Geometry: final body of the model. Coordinates: model frame, mm. A direction names the side the tool comes from. Coordinates: 2 decimals unless noted, no trailing zeros. Order: outer loops, then holes, each group sorted by start corner. A loop starts at its lowest first (then second) coordinate and runs counter-clockwise, first axis right, second up. Notation, with made-up numbers: (5, 37.5) -> (59, 37.5) arc R22 ccw to (59, 70.5) -> close; hole circle Ø10 at (73.5, 81). An arc over 180 degrees is marked (long way). Answer in a Markdown table with one row per item. Add a question column.
1) Set-up query: faces 5 (the face through (9, 1.4, -10)), 6 (the face through (-9.22, 0.71, -10.03)). Return all of +Z, -Z, +X, -X, +Y, -Y with unobstructed straight access to the full face (end or side cutting, diameter ignored); none if empty.
2) Ray query, line 1 (X direction, y = 3.25, z = -9); line 2 (Z direction, x = 12, y = 2.9); line 3 (Z direction, x = 11.5, y = 4.45). Return the intervals inside material, ascending. Write a range as from..to.
3) Section query A-A on x = 0. Return the cut outline in (y, z), then the cut area to 3 significant figures.
4) Pull-direction query (Y, two-part tool) for faces 1 (the face through (0, 0, 0)), 2 (the face through (-9.167, 2.485, 13.124)), 3 (the face through (-9.15, 2.48, 8.1)), 4 (the face through (11.99, 0.71, -10.03)); classes: +Y half, -Y half, draft (parallel to the pull), parting line (faces both ways), or undercut.
5) Section query B-B on y = 4.45. Count the separate pieces of the cut face and the enclosed holes in it, then the cut area to 3 significant figures.
6) Section query C-C on z = 5.5. Return the cut outline in (x, y), then the cut area to 3 significant figures.
7) Contact query for flat-ended pins moving along their axis: P1, Ø3, axis at x = -18, y = 1.5, coming from the +Z side; P2, Ø3, axis at x = -4.5, y = 3.5, coming from the +Z side; P3, Ø2.5, axis at x = 10.61, z = 10.61, coming from the -Y side; P4, Ø6.5, axis at x = -10.5, z = -9.5, coming from the -Y side. Output: stop coordinate, or through.
Autodesk Inventor part; units mm, degrees
ref_plane "Work Plane1" through (0, 2.5, 0) normal (0, 1, 0) x (1, 0, 0)
ref_plane "YZ Plane" through (0, 0, 0) normal (1, 0, 0) x (0, 1, 0)
ref_plane "XZ Plane" through (0, 0, 0) normal (0, 1, 0) x (-1, 0, 0)
sketch "Sketch1" plane through (0, 0, 0) normal (0, 1, 0) x (-1, 0, 0)
  circle A0 centre (0, 0) radius 12.5
  circle A1 centre (12.5, 0) radius 2
  circle A2 centre (0, 12.5) radius 2
  circle A3 centre (-12.5, 0) radius 2
  circle A4 centre (0, -12.5) radius 2
  circle A5 centre (0, 0) radius 22.5
  dimension "d0" = 25
  dimension "d1" = 4
  dimension "d4" = 360
  dimension "d6" = 45
extrude "Extrusion1" add sketch "Sketch1" along normal blind 5 contours A1 A0 A4 A3 A2 | A5
chamfer "Chamfer1" distance 2 angle 45 4 edges at (-10.5, 5, 0) (2, 5, 12.5) (14.5, 5, 0) (2, 5, -12.5)
sketch "Sketch2" plane through (0, 5, 0) normal (0, 1, 0) x (1, 0, 0)
  circle A0 centre (0, 0) radius 15
  line L0 (0, 0) -> (-15, 0)
  line L1 (0, 0) -> (-10.6066, -10.6066)
  circle A1 centre (-10.6066, -10.6066) radius 1.5
  circle A2 centre (10.6066, -10.6066) radius 1.5
  circle A3 centre (10.6066, 10.6066) radius 1.5
  circle A4 centre (-10.6066, 10.6066) radius 1.5
  dimension "d12" = 30
  dimension "d13" = 45
  dimension "d14" = 3
  dimension "d17" = 360
extrude "Extrusion2" cut sketch "Sketch2" against normal blind 5 contours A3 A0 | A0 A3 | A2 A0 | A0 A2 | A4 A0 | A0 A4 | A1 A0 | A0 L1 A1 | A0 A1 L1
ref_plane "Work Plane1" through (0, 2.5, 0) normal (0, 1, 0) x (1, 0, 0)
sketch "Sketch4" plane through (0, 2.5, 0) normal (0, 1, 0) x (1, 0, 0)
  circle A0 centre (10.6066, 10.6066) radius 1.5
  circle A1 centre (10.6066, -10.6066) radius 1.5
  circle A2 centre (-10.6066, -10.6066) radius 1.5
  circle A3 centre (-10.6066, 10.6066) radius 1.5
  line L0 (13.4857, 8.8966) -> (10.5653, 7.2582)
  line L1 (10.5653, 7.2582) -> (7.6862, 8.9682)
  line L2 (7.6862, 8.9682) -> (7.7275, 12.3166)
  line L3 (7.7275, 12.3166) -> (10.6479, 13.955)
  line L4 (10.6479, 13.955) -> (13.527, 12.245)
  line L5 (13.527, 12.245) -> (13.4857, 8.8966)
  point P0 (0, 0)
  dimension "d28" = 5.8
extrude "Extrusion3" cut sketch "Sketch4" along normal mid plane 2.2 contours L0 L1 L2 L3 L4 L5
pattern_circular "Circular Pattern1" count 4 over 360 about axis through (0, 0, 0) along (0, 1, 0) of "Extrusion3"
properties part number "adaptador"
Result:
| question | item | result |
|---|---|---|
| 1 | face 5 | none |
| 1 | face 6 | +Y, -Y |
| 2 | line 1 | -20.62..-13.03, -8.19..7.69, 13.49..20.62 |
| 2 | line 2 | -19.03..-13.15, -8.06..-1.94, 1.94..7.72, 13.52..19.03 |
| 2 | line 3 | -19.34..-11.81, -9.4..-3.3, 3.3..9.4, 11.81..19.34 |
| 3 | outline | (0, -22.5) -> (5, -22.5) -> (5, -16.5) -> (3, -14.5) -> (0, -14.5) -> close; (0, -10.5) -> (3, -10.5) -> (5, -8.5) -> (5, 8.5) -> (3, 10.5) -> (0, 10.5) -> close; (0, 14.5) -> (3, 14.5) -> (5, 16.5) -> (5, 22.5) -> (0, 22.5) -> close |
| 3 | area | 177 mm2 |
| 4 | face 1 | -Y half |
| 4 | face 2 | undercut |
| 4 | face 3 | undercut |
| 4 | face 4 | draft |
| 5 | separate pieces | 1 |
| 5 | enclosed holes | 8 |
| 5 | area | 1,410 mm2 |
| 6 | outline | (-21.82, 0) -> (21.82, 0) -> (21.82, 5) -> (-21.82, 5) -> close |
| 6 | area | 218 mm2 |
| 7 | P1 | z = 15.3 |
| 7 | P2 | z = 22.3 |
| 7 | P3 | through |
| 7 | P4 | y = 0 |
